from build123d import *

# Parameters (mm, degrees)
BOSS_EXTRUDE1_DEPTH = 40
SKETCH3_R           = 13
CUT_EXTRUDE1_DEPTH  = 3
SKETCH4_R           = 1.5
CUT_EXTRUDE2_DEPTH  = 3


with BuildPart() as part:
    # Sketch2 → Boss-Extrude1 (new body)
    with BuildSketch(Plane(origin=(0, 0, 0), x_dir=(0, 0, -1), z_dir=(1, 0, 0))):
        Polygon((0, 0), (22, 0), (22, 42), (20, 42), (20, 2), (0, 2), align=None)
    extrude(amount=BOSS_EXTRUDE1_DEPTH)

    # Sketch3 → Cut-Extrude1 (cut, through all)
    with BuildSketch(Plane.XY.offset(-20)):
        with Locations((20, 21.5)):
            Circle(SKETCH3_R)
    extrude(amount=-CUT_EXTRUDE1_DEPTH, mode=Mode.SUBTRACT)

    # Sketch4 → Cut-Extrude2 (cut, through all)
    with BuildSketch(Plane(origin=(0, 2, 0), x_dir=(1, 0, 0), z_dir=(0, 1, 0))):
        with Locations((35, 5)):
            Circle(SKETCH4_R)
        with Locations((5, 5)):
            Circle(SKETCH4_R)
        with Locations((5, 11)):
            Circle(SKETCH4_R)
        with Locations((5, 17)):
            Circle(SKETCH4_R)
        with Locations((35, 11)):
            Circle(SKETCH4_R)
        with Locations((35, 17)):
            Circle(SKETCH4_R)
    extrude(amount=-CUT_EXTRUDE2_DEPTH, mode=Mode.SUBTRACT)


solid = part.part
Work out the finished part from the listing and answer in its coordinate system (mm). A direction names the side the tool comes from. Coordinates: 2 decimals unless noted, no trailing zeros. Order: outer loops, then holes, each group sorted by start corner. A loop starts at its lowest first (then second) coordinate and runs counter-clockwise, first axis right, second up. Notation, with made-up numbers: (61, 75.25) - (82, 75.25) arc R30 ccw to (82, 108.25) - close; hole circle Ø11 at (62.5, -12.5). An arc over 180 degrees is marked (long way). Put each result on its own line as item: value. Start each with the question number.
1) Find section C-C (y = 21.5). Give the vertices of the cut face in (x, z), plus the area to 3 significant figures.
2) For faces 5 (the flat face through (20, 2, -10)), 6 (the cylindrical face through (6.386, 1.014, -10.425)), determine the directions among +Z, -Z, +X, -X, +Y, -Y from which every point of the face is accessible in a straight line to the end or side of a thin tool.
3) For a pull along Y with two mould halves and no side action, classify faces 1 (the flat face through (20, 0, -11)), 2 (the flat face through (20, 42, -21)), 3 (the flat face through (11, 11, -22)), 4 (the cylindrical face through (26.99, 32.46, -20.99)) as released by +Y, released by -Y, zero draft, split by the parting line, or undercut.
4) Flat-ended cylindrical pins translate along their axes: pin 1 (20 mm diameter, centred on x = 16.5, y = 21, fed in from +Z); pin 2 (5 mm diameter, centred on x = 35, z = -17, fed in from +Y). Find the tip coordinate at first contact, or state that the pin passes through.
5) Find the intervals of material crossed by line 1 (Z direction, x = 35, y = 0.9); line 2 (X direction, y = 1.15, z = -5); line 3 (Y direction, x = 20, z = -20.4), in increasing order. Write a range as from..to.
6) Find section A-A (z = -17). Give the vertices of the cut face in (x, y).
7) Find section D-D (x = 5). Give the vertices of the cut face in (y, z).
8) Find section B-B (x = 20). Give the vertices of the cut face in (y, z).
Results list:
1. outline: (0, -22) - (7, -22) - (7, -20) - (0, -20) - close; (33, -22) - (40, -22) - (40, -20) - (33, -20) - close
1. area: 28.0 mm^2
2. face 5: +Z, +X, -X, +Y
2. face 6: +Y, -Y
3. face 1: released by -Y
3. face 2: released by +Y
3. face 3: zero draft
3. face 4: undercut
4. pin 1: stops at z = -20
4. pin 2: stops at y = 2
5. line 1: z = -22..-18.5, -15.5..-12.5, -9.5..-6.5, -3.5..0
5. line 2: x = 0..3.5, 6.5..33.5, 36.5..40
5. line 3: y = 0..8.5, 34.5..42
6. outline: (0, 0) - (3.5, 0) - (3.5, 2) - (0, 2) - close; (6.5, 0) - (33.5, 0) - (33.5, 2) - (6.5, 2) - close; (36.5, 0) - (40, 0) - (40, 2) - (36.5, 2) - close
7. outline: (0, -22) - (42, -22) - (42, -20) - (2, -20) - (2, -18.5) - (0, -18.5) - close; (0, -15.5) - (2, -15.5) - (2, -12.5) - (0, -12.5) - close; (0, -9.5) - (2, -9.5) - (2, -6.5) - (0, -6.5) - close; (0, -3.5) - (2, -3.5) - (2, 0) - (0, 0) - close
8. outline: (0, -22) - (8.5, -22) - (8.5, -20) - (2, -20) - (2, 0) - (0, 0) - close; (34.5, -22) - (42, -22) - (42, -20) - (34.5, -20) - close
